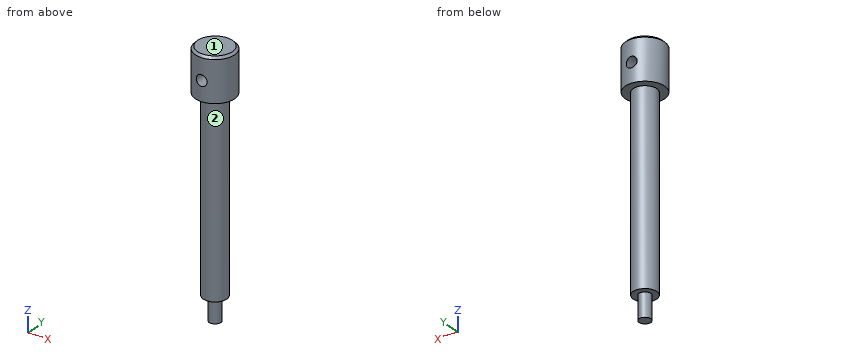
```python
from build123d import *

# Parameters (mm, degrees)
SKETCH3_R               = 10
BOSS_EXTRUDE1_DEPTH     = 22
SKETCH4_R               = 6
BOSS_EXTRUDE2_DEPTH     = 96
SKETCH5_R               = 3
BOSS_EXTRUDE3_DEPTH     = 12
CUT_EXTRUDE2_DEPTH      = 131.766968306
CUT_EXTRUDE2_DEPTH_BACK = 131.766968306
SKETCH6_R               = 2.75
CHAMFER1_SIZE           = 1.15


with BuildPart() as part:
    # Sketch3 → Boss-Extrude1 (new body)
    with BuildSketch(Plane.XY):
        Circle(SKETCH3_R)
    extrude(amount=-BOSS_EXTRUDE1_DEPTH)

    # Sketch4 → Boss-Extrude2 (add)
    with BuildSketch(Plane(origin=(0, 0, -22), x_dir=(-1, 0, 0), z_dir=(0, 0, -1))):
        Circle(SKETCH4_R)
    extrude(amount=BOSS_EXTRUDE2_DEPTH)

    # Sketch5 → Boss-Extrude3 (add)
    with BuildSketch(Plane(origin=(0, 0, -118), x_dir=(-1, 0, 0), z_dir=(0, 0, -1))):
        Circle(SKETCH5_R)
    extrude(amount=BOSS_EXTRUDE3_DEPTH)

    # Sketch6 → Cut-Extrude2 (cut, two sides: drawn at the far end of the back side and taken through both)
    with BuildSketch(Plane(origin=(0, 0, 0), x_dir=(1, 0, 0), z_dir=(0, 1, 0)).offset(-CUT_EXTRUDE2_DEPTH_BACK)):
        with Locations(Location((0, 12, 0), (0, 0, 270))):
            Circle(SKETCH6_R)
    extrude(amount=CUT_EXTRUDE2_DEPTH + CUT_EXTRUDE2_DEPTH_BACK, mode=Mode.SUBTRACT)

    # Chamfer1
    chamfer1_edges = [part.edges().sort_by_distance(p)[0] for p in [
        (-10, 0, 0),
    ]]
    chamfer(chamfer1_edges, length=CHAMFER1_SIZE)


solid = part.part
```
Build history of the part. All positions in model axes, mm. Face numbers are marked on the shaded views. A direction names the side the tool comes from. Round coordinates to 2 decimals unless told otherwise and drop trailing zeros. Write each loop counter-clockwise with the first axis right and the second up, starting at its lowest first coordinate (ties: lowest second). Pieces come first, ordered by that corner, then holes.
1) Band-saw the part on B-B, the plane y = 0. List the corners of the cut face in (x, z), and give its area (3 significant figures).
2) Band-saw the part on A-A, the plane x = 0. List the corners of the cut face in (y, z), and give its area (3 significant figures).
3) Pin check, flat tips, straight feed: pin 1 (10 mm diameter, centred on y = 7.5, z = -49.5, fed in from +X); pin 2 (1.5 mm diameter, centred on y = -8, z = -34.5, fed in from +X); pin 3 (6 mm diameter, centred on x = -3.5, z = -112, fed in from -Y); pin 4 (1 mm diameter, centred on x = 6, y = -1.5, fed in from -Z). Stop position of each tip, or through.
4) Band-saw the part on C-C, the plane z = -12. List the corners of the cut face in (x, y), and give its area (3 significant figures).
5) 3-axis set-ups, long thin cutter, end or side, ignore diameter. For the marked faces 1 and 2: which of +Z, -Z, +X, -X, +Y, -Y reach the whole face in a straight line?
6) Band-saw the part on D-D, the plane z = -109. List the corners of the cut face in (x, y), and give its area (3 significant figures).
7) Drill centre lines: probe 1 along Z at (x, y) = (0, -2.25); probe 2 along Y at (x, z) = (0.25, -9); probe 3 along Z at (x, y) = (0, -4.5). Where is each one in solid material? Low to high.
Ans:
1. outline: (-10, -22) - (-6, -22) - (-6, -118) - (-3, -118) - (-3, -130) - (3, -130) - (3, -118) - (6, -118) - (6, -22) - (10, -22) - (10, -1.15) - (8.85, 0) - (-8.85, 0) - (-10, -1.15) - close; hole circle Ø5.5 at (0, -12)
1. area: 1,640 mm2
2. outline: (-10, -22) - (-6, -22) - (-6, -118) - (-3, -118) - (-3, -130) - (3, -130) - (3, -118) - (6, -118) - (6, -22) - (10, -22) - (10, -14.75) - (-10, -14.75) - close; (-10, -9.25) - (10, -9.25) - (10, -1.15) - (8.85, 0) - (-8.85, 0) - (-10, -1.15) - close
2. area: 1,550 mm2
3. pin 1: stops at x = 5.45
3. pin 2: passes through
3. pin 3: stops at y = -5.98
3. pin 4: stops at z = -118
4. outline: (-2.75, -9.61) - (-2.75, 9.61) arc R10 ccw to start; (2.75, -9.61) arc R10 ccw to (2.75, 9.61) - close
4. area: 206 mm2
5. face 1: +Z, +X, -X, +Y, -Y
5. face 2: -Z
6. outline: circle Ø12 at (0, 0)
6. area: 113 mm2
7. probe 1: z = -130 to -14.75, -9.25 to 0
7. probe 2: y = -10 to 10
7. probe 3: z = -118 to -14.75, -9.25 to 0
